Design review of the part built by this model. Coordinates are the model's own, in mm. Give positions to 0.01 mm unless a question says otherwise; leave off trailing zeros.
from build123d import *

# Parameters (mm, degrees)
F0_W     = 508
F0_H     = 895.35
F1_DEPTH = 19.05
F2_R     = 1.5875
F3_DEPTH = 25.4


with BuildPart() as f1:
    # F0 (on Right) → F1 (new body)
    with BuildSketch(Plane.YZ):
        with Locations((254, 447.675)):
            Rectangle(F0_W, F0_H)
    extrude(amount=F1_DEPTH)

    # F2 (on face) → F3 (cut)
    with BuildSketch(Plane.YZ.offset(19.05)):
        with Locations((88.9, 539.75)):
            Circle(F2_R)
        with Locations((266.7, 539.75)):
            Circle(F2_R)
        with Locations((444.5, 539.75)):
            Circle(F2_R)
    extrude(amount=-F3_DEPTH, mode=Mode.SUBTRACT)


solid = f1.part
Q1. Insertion check: pin 1 (2.5 mm diameter, centred on y = 444.5, z = 539.75, fed in from +X). The pin has a flat end and moves straight along its axis. Give the tip position at first contact, or say it passes through.
Results:
pin 1: passes through
Q2. Wall thickness on line 1 (Y direction, x = 14.75, z = 539.75); line 2 (Z direction, x = 9.5, y = 266.7); line 3 (Z direction, x = 1.25, y = 265.5): over which ranges is each line inside the solid? List them lowest first.
Results:
line 1: y = 0 to 87.31, 90.49 to 265.11, 268.29 to 442.91, 446.09 to 508
line 2: z = 0 to 538.16, 541.34 to 895.35
line 3: z = 0 to 538.71, 540.79 to 895.35
Q3. Draft analysis for pull direction X (two halves, no side actions). For faces 1 (the face through (0, 250, 454)), 2 (the face through (9, 0, 441)), 3 (the face through (19.05, 250, 454)), state which applies: pulls with the +X half, pulls with the -X half, needs draft (parallel to the pull), parting line crosses it, or undercut.
Results:
face 1: pulls with the -X half
face 2: needs draft
face 3: pulls with the +X half
